Autodesk Inventor part; units mm, degrees
ref_plane "YZ Plane" through (0, 0, 0) normal (1, 0, 0) x (0, 1, 0)
ref_plane "XZ Plane" through (0, 0, 0) normal (0, 1, 0) x (-1, 0, 0)
ref_plane "XY Plane" through (0, 0, 0) normal (0, 0, 1) x (1, 0, 0)
sketch "Boceto1" plane through (0, 0, 0) normal (0, 1, 0) x (-1, 0, 0)
  line L0 (0, 0) -> (900, 0)
  line L1 (900, 0) -> (900, -1200)
  line L2 (900, -1200) -> (0, -1200)
  line L3 (0, -1200) -> (0, 0)
  dimension "d0" = 900
  dimension "d1" = 1200
extrude "Extrusión1" add sketch "Boceto1" along normal blind 3
sketch "Boceto2" plane through (0, 3, 0) normal (0, 1, 0) x (1, 0, 0)
  line L0 (0, 1200) -> (-900, 1200)
  line L1 (0, 0) -> (-900, 0)
  line L2 (-900, 0) -> (-900, 1200)
  line L3 (-900, 1200) -> (0, 1200)
  line L4 (0, 1200) -> (0, 0)
  line L5 (-897, 1197) -> (-897, 3)
  line L6 (-897, 3) -> (-3, 3)
  line L7 (-3, 3) -> (-3, 1197)
  line L8 (-3, 1197) -> (-897, 1197)
  dimension "d4" = 3
extrude "Extrusión2" add sketch "Boceto2" along normal blind 50
properties part number "tapa mesa"
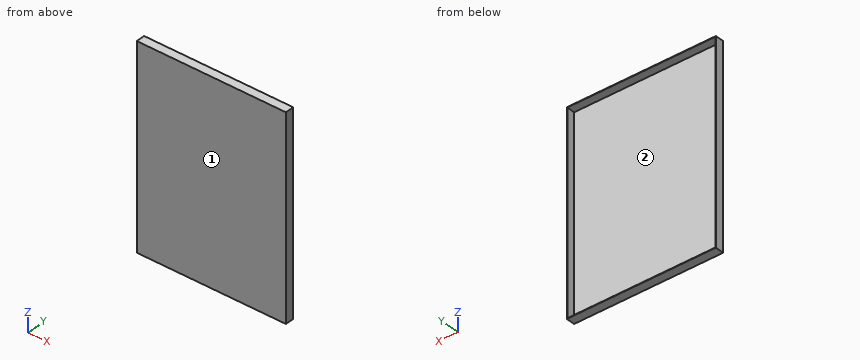
CAD build for the part. Positions are in the model's coordinates, mm. Face numbers are marked on the shaded views. Round coordinates to 2 decimals unless told otherwise and drop trailing zeros. Write each loop counter-clockwise with the first axis right and the second up, starting at its lowest first coordinate (ties: lowest second). Pieces come first, ordered by that corner, then holes. Notation, with made-up numbers: (74.25, 11.25) -> (121.25, 11.25) arc R25 ccw to (121.25, 28.25) -> close; hole circle Ø5 at (-9, -23.5). An arc over 180 degrees is marked (long way). Answer in a Markdown table with one row per item. Add a question column.
Item 1: Saw through at A-A, the plane z = -89.5. Write the cut outline in (x, y).
Item 2: Saw through at C-C, the plane x = -237. Write the cut outline in (y, z), then the cut area to 3 significant figures.
Item 3: Drill centre lines: line 1 (Z direction, x = -701.5, y = 14); line 2 (X direction, y = 24.5, z = -528); line 3 (Y direction, x = -163, z = -988.5). Where is each one in solid material? Low to high. Write a range as from..to.
Item 4: Mould opens along X. For the marked faces 1 and 2 say: pulls with the +X half, pulls with the -X half, needs draft (parallel to the pull), parting line crosses it, or undercut.
Item 5: Drop a flat-ended pin along its axis: pin 1 Ø12 at (x, z) = (-425, -1053) entering from +Y. Give the stop position or say it passes through.
Item 6: Saw through at B-B, the plane y = 36. Write the cut outline in (x, z), then the cut area to 3 significant figures.
Findings below:
| question | item | result |
|---|---|---|
| 1 | outline | (-900, 0) -> (0, 0) -> (0, 53) -> (-3, 53) -> (-3, 3) -> (-897, 3) -> (-897, 53) -> (-900, 53) -> close |
| 2 | outline | (0, -1200) -> (53, -1200) -> (53, -1197) -> (3, -1197) -> (3, -3) -> (53, -3) -> (53, 0) -> (0, 0) -> close |
| 2 | area | 3,900 mm^2 |
| 3 | line 1 | z = -1200..-1197, -3..0 |
| 3 | line 2 | x = -900..-897, -3..0 |
| 3 | line 3 | y = 0..3 |
| 4 | face 1 | needs draft |
| 4 | face 2 | undercut |
| 5 | pin 1 | stops at y = 3 |
| 6 | outline | (-900, -1200) -> (0, -1200) -> (0, 0) -> (-900, 0) -> close; hole (-897, -1197) -> (-3, -1197) -> (-3, -3) -> (-897, -3) -> close |
| 6 | area | 12,600 mm^2 |
